Read the model definition and answer for the solid it produces. Units are mm, in the model's axes. A direction names the side the tool comes from. Give positions to 0.01 mm unless a question says otherwise; leave off trailing zeros. Order: outer loops, then holes, each group sorted by start corner. A loop starts at its lowest first (then second) coordinate and runs counter-clockwise, first axis right, second up.
Item 1: Which of the six approach directions +Z, -Z, +X, -X, +Y, -Y give full straight-line access (tool end or side, diameter ignored) to faces 5 (the face through (-5, 0, 0.5)), 6 (the face through (0, 0, 24)), 7 (the face through (-1.08, -4.88, 12.85))?
Item 2: A cutting plane is placed at D-D (y = 5.5). Write down the section's boundary in (x, z), plus the area to 3 significant figures.
Item 3: Find the intervals of material crossed by line 1 along Z through (x, y) = (1.25, -5.75); line 2 along Z through (x, y) = (0.5, 1.5); line 3 along X through (y, z) = (2.25, 7.5), in increasing order.
Item 4: The mould has two halves that part along X. Classify faces 1 (the face through (3, -1, 0.5)), 2 (the face through (-7.493, 0.33, 0.986)), 3 (the face through (1, -3, 0.5)), 4 (the face through (2, -2, 0)): +X half, -X half, draft (parallel to the pull), parting line (faces both ways), or undercut.
Item 5: Given pin 1 Ø0.5 at (x, z) = (-4, 0.5) entering from -Y; pin 2 Ø2 at (x, z) = (0.5, 10.5) entering from +Y; pin 3 Ø0.8 at (x, z) = (2, 0.5) entering from -Y, each flat-ended and moving along its own axis, determine where each tip first touches the part or whether it passes through.
Item 6: A cutting plane is placed at C-C (z = 3.75). Write down the section's boundary in (x, y), plus the area to 3 significant figures.
Item 7: A cutting plane is placed at A-A (y = 0). Write down the section's boundary in (x, z).
from build123d import *

# Parameters (mm, degrees)
F0_R     = 7.5
F1_DEPTH = 2
F2_R     = 5
F3_DEPTH = 22
F4_W     = 4
F4_H     = 2
F4_W_2   = 2
F4_H_2   = 4
F5_DEPTH = 1


with BuildPart() as f1:
    # F0 (on Top) → F1 (new body)
    with BuildSketch(Plane.XY):
        Circle(F0_R)
    extrude(amount=F1_DEPTH)

    # F2 (on face) → F3 (join)
    with BuildSketch(Plane.XY.offset(2)):
        Circle(F2_R)
    extrude(amount=F3_DEPTH)

    # F4 (on face) → F5 (cut)
    with BuildSketch(Plane(origin=(0, 0, 0), x_dir=(1, 0, 0), z_dir=(0, 0, -1))):
        with Locations((3, 0)):
            Rectangle(F4_W, F4_H)
        with Locations((0, -3)):
            Rectangle(F4_W_2, F4_H_2)
        Rectangle(F4_W_2, F4_H)
        with Locations((-3, 0)):
            Rectangle(F4_W, F4_H)
        with Locations((0, 3)):
            Rectangle(F4_W_2, F4_H_2)
    extrude(amount=-F5_DEPTH, mode=Mode.SUBTRACT)


solid = f1.part
Response values:
1. face 5: -Z
1. face 6: +Z, +X, -X, +Y, -Y
1. face 7: +Z
2. outline: (-5.1, 0) - (5.1, 0) - (5.1, 2) - (-5.1, 2) - close
2. area: 20.4 mm2
3. line 1: z = 0 to 2
3. line 2: z = 1 to 24
3. line 3: x = -4.47 to 4.47
4. face 1: undercut
4. face 2: parting line
4. face 3: undercut
4. face 4: draft
5. pin 1: stops at y = -6.5
5. pin 2: stops at y = 5
5. pin 3: stops at y = -7.33
6. outline: circle Ø10 at (0, 0)
6. area: 78.5 mm2
7. outline: (-7.5, 0) - (-5, 0) - (-5, 1) - (5, 1) - (5, 0) - (7.5, 0) - (7.5, 2) - (5, 2) - (5, 24) - (-5, 24) - (-5, 2) - (-7.5, 2) - close
